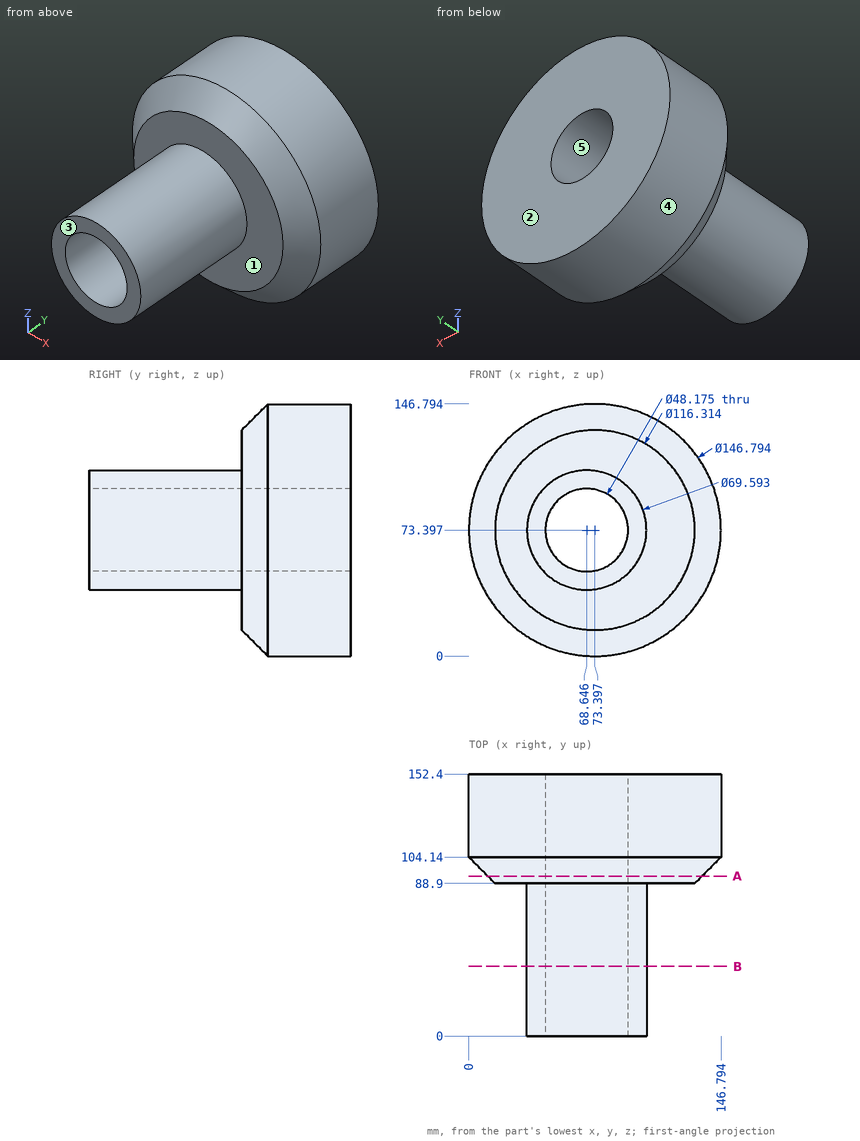
Part print with two shaded views. Sizes in mm from the minimum x, y, z corner. A direction names the side the tool comes from. Coordinates: 2 decimals unless noted, no trailing zeros. Order: outer loops, then holes, each group sorted by start corner. A loop starts at its lowest first (then second) coordinate and runs counter-clockwise, first axis right, second up. Notation, with made-up numbers: M 13,-9.5 L 22,-9.5 A15 cw 22,3.5 Z; hole C 38.25,-24.75 d5. An arc over 180 degrees is marked long. Use a Markdown table: item, result.
(1) Tool access for the marked faces 1 and 2: list every direction of +Z, -Z, +X, -X, +Y, -Y with a clear straight run to the whole face (end or side of a thin tool).
A:
| item | result |
|---|---|
| face 1 | -Y |
| face 2 | +Z, -Z, +X, -X, +Y |
(2) Cut at B-B on y = 40.5. Write the cut outline in (x, z) (1 decimal).
A:
| item | result |
|---|---|
| outline | C 68.6,73.4 d69.6; hole C 68.6,73.4 d48.2 |
(3) Flat gauge pins, fed straight in: pin 1 (1.5 mm diameter, centred on x = 20, y = 121, fed in from -Z) (1 decimal); pin 2 (10 mm diameter, centred on x = 17, z = 55.5, fed in from -Y); pin 3 (3 mm diameter, centred on x = 129.5, y = 116, fed in from -Z). Where does each tip first touch, or does it go through?
A:
| item | result |
|---|---|
| pin 1 | stops at z = 22.3 |
| pin 2 | stops at y = 88.9 |
| pin 3 | stops at z = 24.35 |
(4) Pull direction Z, two halves, no side cores. Call the marked faces 3, 4 and 5: released by +Z, released by -Z, zero draft, split by the parting line, or undercut.
A:
| item | result |
|---|---|
| face 3 | zero draft |
| face 4 | split by the parting line |
| face 5 | undercut |
(5) Cut at A-A on y = 93. Write the cut outline in (x, z) (1 decimal), then the cut area to 3 significant figures.
A:
| item | result |
|---|---|
| outline | C 73.4,73.4 d124.5; hole C 68.6,73.4 d48.2 |
| area | 10,400 mm^2 |
(6) Probe L1, parallel to Z at x = 64, y = 89 (1 decimal); L2, parallel to Y at x = 19.5, z = 86.5; L3, parallel to X at y = 53, z = 57 (1 decimal). List the from-to ranges inside material, lowest first.
A:
| item | result |
|---|---|
| L1 | z = 15.9 to 49.8, 97 to 130.9 |
| L2 | y = 88.9 to 152.4 |
| L3 | x = 38 to 51, 86.3 to 99.3 |
